```python
from build123d import *

# Parameters (mm, degrees)
F0_R     = 8.05
F1_DEPTH = 3
F2_W     = 10
F2_H     = 3
F3_DEPTH = 3
F4_DEPTH = 9
F5_W     = 10
F5_H     = 3
F6_DEPTH = 40


with BuildPart() as f1:
    # F0 (on Top) → F1 (new body)
    with BuildSketch(Plane.XY):
        with BuildLine():
            ThreePointArc((-3.5381985419, -8.9346590881), (-0.9167500432, -4.8048668541), (0, 0))
            ThreePointArc((0, 0), (-0.9167500432, 4.8048668541), (-3.5381985419, 8.9346590881))
            ThreePointArc((-3.5381985419, 8.9346590881), (-26.1, 0), (-3.5381985419, -8.9346590881))
        make_face()
        with Locations((-13.05, 0)):
            Circle(F0_R, mode=Mode.SUBTRACT)
        with BuildLine():
            Line((0, -9.6097337082), (0, 0))
            ThreePointArc((0, 0), (-0.9167500432, -4.8048668541), (-3.5381985419, -8.9346590881))
            ThreePointArc((-3.5381985419, -8.9346590881), (-1.8010118451, -9.4394564609), (0, -9.6097337082))
        make_face()
        with BuildLine():
            ThreePointArc((-3.5381985419, 8.9346590881), (-0.9167500432, 4.8048668541), (0, 0))
            Line((0, 0), (0, 9.6097337082))
            ThreePointArc((0, 9.6097337082), (-1.8010118451, 9.4394564609), (-3.5381985419, 8.9346590881))
        make_face()
    extrude(amount=F1_DEPTH)

    # F2 (on face) → F3 (join, through all)
    with BuildSketch(Plane(origin=(0, 0, 0), x_dir=(1, 0, 0), z_dir=(0, 0, -1))):
        with BuildLine():
            ThreePointArc((-18.05, 12.0541486634), (-13.05, 13.05), (-8.05, 12.0541486634))
            Line((-8.05, 12.0541486634), (-8.05, 15.45))
            Line((-8.05, 15.45), (-18.05, 15.45))
            Line((-18.05, 15.45), (-18.05, 12.0541486634))
        make_face()
        with Locations((-13.05, 16.95)):
            Rectangle(F2_W, F2_H)
    extrude(amount=-F3_DEPTH)

    # F2 (on face) → F4 (join)
    with BuildSketch(Plane(origin=(0, 0, 0), x_dir=(1, 0, 0), z_dir=(0, 0, -1))):
        with Locations((-13.05, 16.95)):
            Rectangle(F2_W, F2_H)
    extrude(amount=F4_DEPTH)

    # F5 (on face) → F6 (join)
    with BuildSketch(Plane.XZ.offset(18.45)):
        with Locations((-13.05, -10.5)):
            Rectangle(F5_W, F5_H)
    extrude(amount=-F6_DEPTH)

    # F7: F1 across plane


with BuildPart() as f1_1:
    add(f1.part)
    add(f1.part.mirror(Plane.YZ))


solid = f1_1.part
```
The listing builds one solid part. Answer for the finished solid, in the listing's coordinates (mm). A direction names the side the tool comes from. Give positions to 0.01 mm unless a question says otherwise; leave off trailing zeros. Order: outer loops, then holes, each group sorted by start corner. A loop starts at its lowest first (then second) coordinate and runs counter-clockwise, first axis right, second up.
1) Find section B-B on y = 0. Write down the section's boundary in (x, z).
Reported:
outline: (-26.1, 0) - (-21.1, 0) - (-21.1, 3) - (-26.1, 3) - close; (-18.05, -12) - (-8.05, -12) - (-8.05, -9) - (-18.05, -9) - close; (-5, 0) - (5, 0) - (5, 3) - (-5, 3) - close; (8.05, -12) - (18.05, -12) - (18.05, -9) - (8.05, -9) - close; (21.1, 0) - (26.1, 0) - (26.1, 3) - (21.1, 3) - close
2) Find section A-A on x = -13.05. Write down the section's boundary in (y, z), then the cut area to 3 significant figures.
Reported:
outline: (-18.45, -12) - (21.55, -12) - (21.55, -9) - (-15.45, -9) - (-15.45, 0) - (-8.05, 0) - (-8.05, 3) - (-18.45, 3) - close; (8.05, 0) - (13.05, 0) - (13.05, 3) - (8.05, 3) - close
area: 193 mm2
3) Given P1, Ø8, axis at x = 13.5, y = 0, coming from the +Z side; P2, Ø1.5, axis at x = -6, y = 5, coming from the -Z side; P3, Ø7, axis at x = 14.5, z = -3, coming from the +Y side, each flat-ended and moving along its own axis, determine where each tip first touches the part or whether it passes through.
Reported:
P1: stops at z = -9
P2: stops at z = 0
P3: stops at y = 13.05
4) Consider line 1 along Y through (x, z) = (-13.05, 0.9); line 2 along Z through (x, y) = (-13.5, 12); line 3 along X through (y, z) = (-16, -3.25). Determine where each line is inside the solid, lowest interval first.
Reported:
line 1: y = -18.45 to -8.05, 8.05 to 13.05
line 2: z = -12 to -9, 0 to 3
line 3: x = -18.05 to -8.05, 8.05 to 18.05
5) Find section C-C on z = -2. Write down the section's boundary in (x, y), then the cut area to 3 significant figures.
Reported:
outline: (-18.05, -18.45) - (-8.05, -18.45) - (-8.05, -15.45) - (-18.05, -15.45) - close; (8.05, -18.45) - (18.05, -18.45) - (18.05, -15.45) - (8.05, -15.45) - close
area: 60.0 mm2
6) Find section D-D on y = 17.5. Write down the section's boundary in (x, z), then the cut area to 3 significant figures.
Reported:
outline: (-18.05, -12) - (-8.05, -12) - (-8.05, -9) - (-18.05, -9) - close; (8.05, -12) - (18.05, -12) - (18.05, -9) - (8.05, -9) - close
area: 60.0 mm2
7) Determine the mould class of faces 1 (the face through (0, -2, 3)), 2 (the face through (-18.05, -3, -10)), 3 (the face through (-5.372, 2.418, 1.479)) for opening direction X: pulls with the +X half, pulls with the -X half, needs draft (parallel to the pull), parting line crosses it, or undercut.
Reported:
face 1: needs draft
face 2: pulls with the -X half
face 3: undercut
8) For faces 4 (the face through (0, -1, 0)), 5 (the face through (-5.66, -10.756, 1.479)), 6 (the face through (-23.596, 7.687, 1.479)), determine the directions among +Z, -Z, +X, -X, +Y, -Y from which every point of the face is accessible in a straight line to the end or side of a thin tool.
Reported:
face 4: +X, -X, +Y
face 5: +Z, -Z, -Y
face 6: +Z
